Could you check a few things on this model? Use its own coordinates, in mm. A direction names the side the tool comes from. Give positions to 0.01 mm unless a question says otherwise; leave off trailing zeros. Order: outer loops, then holes, each group sorted by start corner. A loop starts at its lowest first (then second) coordinate and runs counter-clockwise, first axis right, second up.
(1) Imagine slicing it at D-D, the plane z = 3. Write out the boundary of the cut face in (x, y), then the cut area to 3 significant figures.
(2) Imagine slicing it at C-C, the plane x = 35. Write out the boundary of the cut face in (y, z), then the cut area to 3 significant figures.
(3) On a 3-axis mill with a long thin cutter (end or side, diameter ignored), from which of +Z, -Z, +X, -X, +Y, -Y can I reach the whole of each face in a straight line? I mean faces 5 (the cylindrical face through (33.8, 6.5, 5.1)), 6 (the flat face through (25, 3, 10)). Say none if no direction works.
(4) Will these pins go through, and if not, where does the flat tip stop? pin 1 (17 mm diameter, centred on x = 29.5, z = 7.5, fed in from -Y); pin 2 (0.9 mm diameter, centred on y = 1.5, z = 10.5, fed in from +X); pin 3 (1 mm diameter, centred on x = 23, y = 3, fed in from -Z); pin 4 (2.5 mm diameter, centred on x = 15, z = 6, fed in from -Y).
(5) If I drill on probe 1 along Z at (x, y) = (15, 5.75); probe 2 along Z at (x, y) = (16, 5.25); probe 3 along Y at (x, z) = (21.5, 18), over which ranges is the centre line in solid material (lowest first)?
(6) Imagine slicing it at B-B, the plane y = 9. Write out the boundary of the cut face in (x, z), then the cut area to 3 significant figures.
(7) If we mould it in two halves opening along Z, with no side actions, what happens to faces 1 (the flat face through (20, 6, 0)), 2 (the cylindrical face through (13.5, 6.45, 6.07)), 3 (the flat face through (2, 2, 26)), 4 (the cylindrical face through (13.5, 6.45, 15.07))? For each: released by +Z, released by -Z, zero draft, split by the parting line, or undercut.
(8) Imagine slicing it at A-A, the plane z = 15. Write out the boundary of the cut face in (x, y).
from build123d import *

# Parameters (mm, degrees)
PAD_DEPTH         = 21
SKETCH001_R       = 2
PAD001_DEPTH      = 5
PAD001_DEPTH_BACK = 26
SKETCH002_R       = 1.5
POCKET_DEPTH      = 7.001


with BuildPart() as part:
    # Sketch → Pad (new body)
    with BuildSketch(Plane.XY):
        with BuildLine():
            Line((0, 10), (40, 10))
            Line((40, 10), (40, 3))
            Line((40, 3), (10, 3))
            Line((10, 3), (10, 0))
            Line((10, 0), (2, 0))
            ThreePointArc((0, 2), (0.585786, 0.585786), (2, 0))
            Line((0, 10), (0, 2))
        make_face()
    extrude(amount=PAD_DEPTH)

    # Sketch001 → Pad001 (new body, two sides)
    with BuildSketch(Plane(origin=(0, 0, 0), x_dir=(1, 0, 0), z_dir=(0, 0, -1))) as pad001_sk:
        with Locations((2, -2)):
            Circle(SKETCH001_R)
    extrude(amount=PAD001_DEPTH)
    extrude(pad001_sk.sketch, amount=-PAD001_DEPTH_BACK)

    # Sketch002 → Pocket (cut, through all)
    with BuildSketch(Plane.XZ.offset(-3)):
        with Locations((15, 15)):
            Circle(SKETCH002_R)
        with Locations((35, 15)):
            Circle(SKETCH002_R)
        with Locations((15, 6)):
            Circle(SKETCH002_R)
        with Locations((35, 6)):
            Circle(SKETCH002_R)
    extrude(amount=-POCKET_DEPTH, mode=Mode.SUBTRACT)


solid = part.part
Answer block:
1. outline: (0, 2) arc R2 ccw to (2, 0) - (10, 0) - (10, 3) - (40, 3) - (40, 10) - (0, 10) - close
1. area: 309 mm2
2. outline: (3, 0) - (10, 0) - (10, 4.5) - (3, 4.5) - close; (3, 7.5) - (10, 7.5) - (10, 13.5) - (3, 13.5) - close; (3, 16.5) - (10, 16.5) - (10, 21) - (3, 21) - close
2. area: 105 mm2
3. face 5: +Y, -Y
3. face 6: +Z, -Z, +X, -Y
4. pin 1: stops at y = 3
4. pin 2: stops at x = 10
4. pin 3: stops at z = 0
4. pin 4: passes through
5. probe 1: z = 0 to 4.5, 7.5 to 13.5, 16.5 to 21
5. probe 2: z = 0 to 4.88, 7.12 to 13.88, 16.12 to 21
5. probe 3: y = 3 to 10
6. outline: (0, 0) - (40, 0) - (40, 21) - (0, 21) - close; hole circle Ø3 at (15, 6); hole circle Ø3 at (15, 15); hole circle Ø3 at (35, 6); hole circle Ø3 at (35, 15)
6. area: 812 mm2
7. face 1: released by -Z
7. face 2: undercut
7. face 3: released by +Z
7. face 4: undercut
8. outline: (0, 2) arc R2 ccw to (2, 0) - (10, 0) - (10, 3) - (13.5, 3) - (13.5, 10) - (0, 10) - close; (16.5, 3) - (33.5, 3) - (33.5, 10) - (16.5, 10) - close; (36.5, 3) - (40, 3) - (40, 10) - (36.5, 10) - close
